Could you check a few things on this model? Use its own coordinates, in mm. A direction names the side the tool comes from. Give positions to 0.01 mm unless a question says otherwise; leave off trailing zeros. Loops run counter-clockwise (first coordinate to the right, second up) from the corner with the lowest first, then second, coordinate; pieces in that order, holes last. Notation, with made-up numbers: (62.25, 4) - (73.25, 4) arc R31 ccw to (73.25, 43) - close; hole circle Ø1 at (-0.5, 83). An arc over 180 degrees is marked (long way). Use CSV: the item, a comma, the result in double quotes.
from build123d import *

# Parameters (mm, degrees)
F0_R      = 6.5
F1_DEPTH  = 33.3
F2_SIZE   = 3
F3_W      = 27
F3_H      = 12
F4_DEPTH  = 2
F5_R      = 1
F6_DEPTH  = 8
F7_R      = 0.8
F8_R      = 1.5
F8_R_2    = 1.3212801888
F9_DEPTH  = 25
F11_DEPTH = 2
F12_W     = 9
F12_H     = 44.6074357137
F13_DEPTH = 5
F14_W     = 9
F14_H     = 35.2907052629
F15_DEPTH = 5


with BuildPart() as f1:
    # F0 (on Top) → F1 (new body)
    with BuildSketch(Plane.XY):
        Circle(F0_R)
    extrude(amount=F1_DEPTH)

    # F2
    f2_edges = [f1.edges().sort_by_distance(p)[0] for p in [
        (-6.5, 0, 0),
    ]]
    chamfer(f2_edges, length=F2_SIZE)

    # F3 (on face) → F4 (join)
    with BuildSketch(Plane.XY.offset(33.3)):
        Rectangle(F3_W, F3_H)
    extrude(amount=F4_DEPTH)

    # F5 (on face) → F6 (join)
    with BuildSketch(Plane(origin=(0, 0, 0), x_dir=(1, 0, 0), z_dir=(0, 0, -1))):
        Circle(F5_R)
    extrude(amount=F6_DEPTH)

    # F7
    f7_edges = [f1.edges().sort_by_distance(p)[0] for p in [
        (-1, 0, -8),
    ]]
    fillet(f7_edges, radius=F7_R)

    # F8 (on face) → F9 (cut)
    with BuildSketch(Plane.XY.offset(35.3)):
        with Locations((-9, 0)):
            Circle(F8_R)
        with Locations((9, 0)):
            Circle(F8_R_2)
    extrude(amount=-F9_DEPTH, mode=Mode.SUBTRACT)

    # F10 (on face) → F11 (cut, through all)
    with BuildSketch(Plane.XY.offset(35.3)):
        Polygon((-13.5, -4), (-13.5, -6), (-4.5, -6), align=None)
        Polygon((-4.5, 6), (-13.5, 6), (-13.5, 4), align=None)
        Polygon((13.5, -4), (4.5, -6), (13.5, -6), align=None)
        Polygon((13.5, 4), (13.5, 6), (4.5, 6), align=None)
    extrude(amount=-F11_DEPTH, mode=Mode.SUBTRACT)

    # F12 (on face) → F13 (cut)
    with BuildSketch(Plane.XZ.offset(6)):
        with Locations((0, 12.9962821431)):
            Rectangle(F12_W, F12_H)
    extrude(amount=F13_DEPTH, mode=Mode.SUBTRACT)

    # F14 (on face) → F15 (cut)
    with BuildSketch(Plane(origin=(0, 6, 0), x_dir=(-1, 0, 0), z_dir=(0, 1, 0))):
        with Locations((0, 15.6546473686)):
            Rectangle(F14_W, F14_H)
    extrude(amount=F15_DEPTH, mode=Mode.SUBTRACT)


solid = f1.part
1) I need wall thicknesses on line 1 along X through (y, z) = (0, 21); line 2 along Y through (x, z) = (-9, 34.6); line 3 along X through (y, z) = (2.5, 13). Which ranges of each line are inside material? Lowest first, please.
Answer below:
line 1,"x = -6.5 to 6.5"
line 2,"y = -5 to -1.5, 1.5 to 5"
line 3,"x = -6 to 6"
2) I'm going to push flat-ended pins straight in: P1, Ø2.5, axis at x = -9, y = 0, coming from the +Z side; P2, Ø5.5, axis at x = -8.5, y = 0, coming from the -Z side; P3, Ø2, axis at y = 4, z = 9, coming from the +X side; P4, Ø1, axis at y = 1, z = 17.5, coming from the -X side. Where does each tip first touch, or does it pass through?
Answer below:
P1,"passes through"
P2,"stops at z = 2.25"
P3,"stops at x = 5.77"
P4,"stops at x = -6.48"
3) Suppose I cut it at A-A (x = -9). Please give me the cut outline in (y, z).
Answer below:
outline,"(-5, 33.3) - (-1.5, 33.3) - (-1.5, 35.3) - (-5, 35.3) - close; (1.5, 33.3) - (5, 33.3) - (5, 35.3) - (1.5, 35.3) - close"
4) Suppose I cut it at C-C (z = -3.5). Please give me the cut outline in (x, y), plus the area to 3 significant figures.
Answer below:
outline,"circle Ø2 at (0, 0)"
area,"3.14 mm2"
5) Which directions (+Z, -Z, +X, -X, +Y, -Y) give clear straight access to the entire face, cutting with the end or side of a thin tool? Please do faces 1 (the cylindrical face through (-6.5, 0.1, 17.9)), 2 (the flat face through (1, -1, 0)), 3 (the cylindrical face through (6.5, -0.1, 17.9)).
Answer below:
face 1,"-Z, -X"
face 2,"-Z"
face 3,"-Z, +X"
6) Suppose I cut it at D-D (z = 12.5). Please give me the cut outline in (x, y).
Answer below:
outline,"(-2.5, -6) - (2.5, -6) arc R6.5 ccw to (2.5, 6) - (-2.5, 6) arc R6.5 ccw to start"
7) We'd pull the mould along X, two halves only. Please class faces 4 (the cylindrical face through (-10.5, 0.07, 34.31)), 5 (the flat face through (0, -6, 19)), 6 (the conical face through (3.48, 1.1, 0.15)): +X half, -X half, draft (parallel to the pull), parting line (faces both ways), or undercut.
Answer below:
face 4,"undercut"
face 5,"draft"
face 6,"parting line"
8) Suppose I cut it at B-B (x = 9). Please give me the cut outline in (y, z), plus the area to 3 significant figures.
Answer below:
outline,"(-5, 33.3) - (-1.32, 33.3) - (-1.32, 35.3) - (-5, 35.3) - close; (1.32, 33.3) - (5, 33.3) - (5, 35.3) - (1.32, 35.3) - close"
area,"14.7 mm2"
